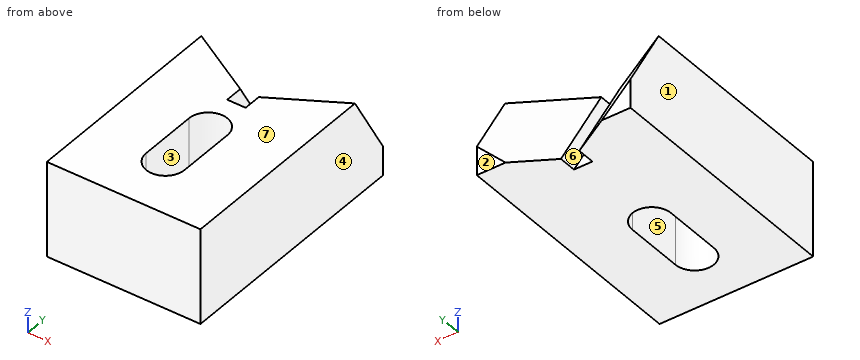
```python
from build123d import *

# Parameters (mm, degrees)
SKETCH1_W           = 50.8
SKETCH1_H           = 82.296
BOSS_EXTRUDE1_DEPTH = 31.496
CUT_EXTRUDE1_DEPTH  = 37.523148695


with BuildPart() as part:
    # Sketch1 → Boss-Extrude1 (new body)
    with BuildSketch(Plane.XY):
        with Locations((0, 41.148)):
            Rectangle(SKETCH1_W, SKETCH1_H)
        with BuildLine():
            Line((6.35, 38.1), (6.35, 18.796))
            ThreePointArc((6.35, 18.796), (0, 12.446), (-6.35, 18.796))
            Line((-6.35, 18.796), (-6.35, 38.1))
            ThreePointArc((-6.35, 38.1), (0, 44.45), (6.35, 38.1))
        make_face(mode=Mode.SUBTRACT)
    extrude(amount=BOSS_EXTRUDE1_DEPTH)

    # Sketch2 → Cut-Extrude1 (cut, through all, along a direction that is not the sketch's normal)
    with BuildSketch(Plane.XY.offset(31.496)):
        Polygon((-25.4, 69.596), (-3.048, 56.691066783), (-3.048, 50.8), (3.048, 50.8), (3.048, 56.691066783), (25.4, 69.596), (25.4, 82.296), (-25.4, 82.296), align=None)
    extrude(amount=-CUT_EXTRUDE1_DEPTH, dir=(0, -0.5, 0.866025404), mode=Mode.SUBTRACT)


solid = part.part
```
Design review of the part built by this model. Coordinates are the model's own, in mm. Face numbers are marked on the shaded views. A direction names the side the tool comes from. Coordinates: 2 decimals unless noted, no trailing zeros. Loops run counter-clockwise (first coordinate to the right, second up) from the corner with the lowest first, then second, coordinate; pieces in that order, holes last. Notation, with made-up numbers: (14.5, 61) -> (29.5, 61) arc R8 cw to (29.5, 68) -> close; hole circle Ø1 at (14, 55.5). An arc over 180 degrees is marked (long way). Answer as a JSON object with one key per item and string values.
Q1. To check wall thickness, follow L1, parallel to X at y = 31, z = 18; L2, parallel to Y at x = 1.5, z = 2.5. State the ranges of each line that lie inside material, in increasing order.
Answer block:
{"L1": "x = -25.4 to -6.35, 6.35 to 25.4", "L2": "y = 0 to 12.63, 44.27 to 67.54"}
Q2. Take a section at B-B on z = 4. Give the boundary of the cut face in (x, y), plus the area to 3 significant figures.
Answer block:
{"outline": "(-25.4, 0) -> (25.4, 0) -> (25.4, 82.3) -> (19.9, 82.3) -> (3.05, 72.57) -> (3.05, 66.67) -> (-3.05, 66.67) -> (-3.05, 72.57) -> (-19.9, 82.3) -> (-25.4, 82.3) -> close; hole (-6.35, 18.8) arc R6.35 ccw to (6.35, 18.8) -> (6.35, 38.1) arc R6.35 ccw to (-6.35, 38.1) -> close", "area": "3,550 mm^2"}
Q3. Clearance check with flat-ended pins moving along their axes: pin 1 Ø6 at (x, z) = (9.5, 7.5) entering from +Y; pin 2 Ø8 at (x, z) = (3.5, 24.5) entering from +Y. State where each tip first meets the part, or that it passes through.
Answer block:
{"pin 1": "stops at y = 76.72", "pin 2": "stops at y = 64.26"}
Q4. Take a section at C-C on y = 54. Give the boundary of the cut face in (x, z), plus the area to 3 significant figures.
Answer block:
{"outline": "(-25.4, 0) -> (25.4, 0) -> (25.4, 31.5) -> (3.05, 31.5) -> (3.05, 25.95) -> (-3.05, 25.95) -> (-3.05, 31.5) -> (-25.4, 31.5) -> close", "area": "1,570 mm^2"}
Q5. Take a section at D-D on x = -8. Give the boundary of the cut face in (y, z).
Answer block:
{"outline": "(0, 0) -> (77.73, 0) -> (59.55, 31.5) -> (0, 31.5) -> close"}
Q6. The part is to be moulded in two halves that separate along X. For the marked faces 1, 2, 3 and 4, say which applies: +X half, -X half, draft (parallel to the pull), parting line (faces both ways), or undercut.
Answer block:
{"face 1": "-X half", "face 2": "draft", "face 3": "undercut", "face 4": "+X half"}
Q7. Take a section at A-A on x = 0. Give the boundary of the cut face in (y, z), plus the area to 3 significant figures.
Answer block:
{"outline": "(0, 0) -> (12.45, 0) -> (12.45, 31.5) -> (0, 31.5) -> close; (44.45, 0) -> (68.98, 0) -> (50.8, 31.5) -> (44.45, 31.5) -> close", "area": "878 mm^2"}
Q8. Tool access review of the marked faces 5, 6 and 7: name each direction out of +Z, -Z, +X, -X, +Y, -Y from which nothing blocks a thin tool from reaching the whole face with its end or side.
Answer block:
{"face 5": "+Z, -Z", "face 6": "+Z, +Y", "face 7": "+Z, +X, -X, +Y, -Y"}
